```python
from build123d import *

# Parameters (mm, degrees)
CROQUIS1_R              = 7
CROQUIS1_R_2            = 4
SALIENTE_EXTRUIR1_DEPTH = 32
CROQUIS2_R              = 4
SALIENTE_EXTRUIR2_DEPTH = 3
CROQUIS3_R              = 5.5
SALIENTE_EXTRUIR3_DEPTH = 1
CROQUIS4_R              = 6
SALIENTE_EXTRUIR4_DEPTH = 8
CROQUIS5_R              = 2
CORTAR_EXTRUIR1_DEPTH   = 34
CHAFL_N1_SIZE           = 3
CHAFL_N1_SIZE2          = 2.100622615
CHAFL_N2_SIZE           = 0.5
CHAFL_N2_SIZE2          = 0.419549816
CHAFL_N3_SIZE           = 0.5
CHAFL_N3_SIZE2          = 0.419549816
CROQUIS6_R              = 5.5
CROQUIS6_R_2            = 4
SALIENTE_EXTRUIR5_DEPTH = 4


with BuildPart() as part:
    # Croquis1 → Saliente-Extruir1 (new body)
    with BuildSketch(Plane(origin=(0, 0, 0), x_dir=(1, 0, 0), z_dir=(0, 1, 0))):
        Circle(CROQUIS1_R)
        Circle(CROQUIS1_R_2, mode=Mode.SUBTRACT)
    extrude(amount=SALIENTE_EXTRUIR1_DEPTH)

    # Croquis2 → Saliente-Extruir2 (add)
    with BuildSketch(Plane(origin=(0, 3, 0), x_dir=(1, 0, 0), z_dir=(0, 1, 0))):
        Circle(CROQUIS2_R)
    extrude(amount=-SALIENTE_EXTRUIR2_DEPTH)

    # Croquis3 → Saliente-Extruir3 (add)
    with BuildSketch(Plane(origin=(0, 0, 0), x_dir=(-1, 0, 0), z_dir=(0, -1, 0))):
        Circle(CROQUIS3_R)
    extrude(amount=SALIENTE_EXTRUIR3_DEPTH)

    # Croquis4 → Saliente-Extruir4 (add)
    with BuildSketch(Plane.XZ.offset(1)):
        Circle(CROQUIS4_R)
    extrude(amount=SALIENTE_EXTRUIR4_DEPTH)

    # Croquis5 → Cortar-Extruir1 (cut)
    with BuildSketch(Plane.XZ.offset(9)):
        Circle(CROQUIS5_R)
    extrude(amount=-CORTAR_EXTRUIR1_DEPTH, mode=Mode.SUBTRACT)

    # Chaflán1
    chafl_n1_edges = [part.edges().sort_by_distance(p)[0] for p in [
        (-2, -9, 0),
    ]]
    chafl_n1_side = [part.faces().sort_by_distance(p)[0] for p in [
        (-5.830294373, -9, 0),
    ]]
    chamfer(chafl_n1_edges, length=CHAFL_N1_SIZE, length2=CHAFL_N1_SIZE2, reference=chafl_n1_side[0])

    # Chaflán2
    chafl_n2_edges = [part.edges().sort_by_distance(p)[0] for p in [
        (-6, -9, 0),
    ]]
    chafl_n2_side = [part.faces().sort_by_distance(p)[0] for p in [
        (-6, -5, 0),
    ]]
    chamfer(chafl_n2_edges, length=CHAFL_N2_SIZE, length2=CHAFL_N2_SIZE2, reference=chafl_n2_side[0])

    # Chaflán3
    chafl_n3_edges = [part.edges().sort_by_distance(p)[0] for p in [
        (-7, 32, 0),
    ]]
    chafl_n3_side = [part.faces().sort_by_distance(p)[0] for p in [
        (-7, 16, 0),
    ]]
    chamfer(chafl_n3_edges, length=CHAFL_N3_SIZE, length2=CHAFL_N3_SIZE2, reference=chafl_n3_side[0])

    # Croquis6 → Saliente-Extruir5 (add)
    with BuildSketch(Plane(origin=(0, 32, 0), x_dir=(1, 0, 0), z_dir=(0, 1, 0))):
        Circle(CROQUIS6_R)
        Circle(CROQUIS6_R_2, mode=Mode.SUBTRACT)
    extrude(amount=SALIENTE_EXTRUIR5_DEPTH)


solid = part.part
```
Design review of the part built by this model. Coordinates are the model's own, in mm. A direction names the side the tool comes from. Coordinates: 2 decimals unless noted, no trailing zeros. Order: outer loops, then holes, each group sorted by start corner. A loop starts at its lowest first (then second) coordinate and runs counter-clockwise, first axis right, second up.
1) For faces 4 (the cylindrical face through (-6, -5, 0)), 5 (the flat face through (-4, 36, 2)), 6 (the cylindrical face through (-0.867, 19.269, 3.905)), 7 (the cylindrical face through (1.19, -0.49, 5.37)), list the 3-axis set-ups (+Z, -Z, +X, -X, +Y, -Y) from which the entire face can be reached by the end or side of a thin tool; tool diameter is ignored.
2) Mouldability with a two-part tool opening along X and no side actions: class faces 1 (the flat face through (-5, -9, 2)), 2 (the cylindrical face through (0, -2, -2)), 3 (the cylindrical face through (6.466, 15.53, 2.681)) as +X half, -X half, draft (parallel to the pull), parting line (faces both ways), or undercut.
3) Take a section at C-C, the plane y = 20. Give the boundary of the cut face in (x, z).
4) Wall thickness on line 1 along Z through (x, y) = (0, -4); line 2 along X through (y, z) = (21, 0): over which ranges is each line inside the solid? List them lowest first.
5) Clearance check with flat-ended pins moving along their axes: pin 1 (2 mm diameter, centred on x = 5, y = 13.5, fed in from +Z); pin 2 (3.5 mm diameter, centred on x = 0, z = 0, fed in from -Y); pin 3 (5 mm diameter, centred on x = 3, y = 24, fed in from -Z); pin 4 (6.5 mm diameter, centred on x = 0, z = 0, fed in from -Y). State where each tip first meets the part, or that it passes through.
Returned:
1. face 4: -Y
1. face 5: +Z, -Z, +X, -X, +Y
1. face 6: +Y
1. face 7: none
2. face 1: draft
2. face 2: undercut
2. face 3: parting line
3. outline: circle Ø14 at (0, 0); hole circle Ø8 at (0, 0)
4. line 1: z = -6 to -2, 2 to 6
4. line 2: x = -7 to -4, 4 to 7
5. pin 1: stops at z = 5.74
5. pin 2: passes through
5. pin 3: stops at z = -6.98
5. pin 4: stops at y = -7.77
